Autodesk Inventor part; units mm, degrees
ref_plane "YZ Plane" through (0, 0, 0) normal (1, 0, 0) x (0, 1, 0)
ref_plane "XZ Plane" through (0, 0, 0) normal (0, 1, 0) x (-1, 0, 0)
ref_plane "XY Plane" through (0, 0, 0) normal (0, 0, 1) x (1, 0, 0)
sketch "Sketch1" plane through (0, 0, 0) normal (0, 1, 0) x (-1, 0, 0)
  circle A0 centre (0, 0) radius 3
  circle A1 centre (0, 0) radius 11.049
  circle A2 centre (0, -7.9375) radius 1.27
  circle A3 centre (7.9375, 0) radius 1.27
  circle A4 centre (0, 7.9375) radius 1.27
  circle A5 centre (-7.9375, 0) radius 1.27
  dimension "d4" = 6
  dimension "d6" = 22.098
  dimension "d10" = 2.54
  dimension "d11" = 7.9375
  dimension "d14" = 360
extrude "Extrusion1" add sketch "Sketch1" along normal mid plane 6.35
sketch "Sketch2" plane through (0, 3.175, 0) normal (0, 1, 0) x (1, 0, 0)
  circle A0 centre (0, 0) radius 3
  circle A1 centre (0, 0) radius 4.699
  dimension "d18" = 6
  dimension "d19" = 9.398
extrude "Extrusion2" add sketch "Sketch2" along normal blind 3.175
sketch "Sketch3" plane through (0, -3.175, 0) normal (0, -1, 0) x (1, 0, 0)
  circle A0 centre (0, 0) radius 3
  circle A1 centre (0, 0) radius 4.699
  dimension "d22" = 6
  dimension "d23" = 9.398
extrude "Extrusion3" add sketch "Sketch3" along normal blind 3.175
properties part number "CouplingScrew"
Design review of the part built by this model. Coordinates are the model's own, in mm. A direction names the side the tool comes from. Coordinates: 2 decimals unless noted, no trailing zeros. Order: outer loops, then holes, each group sorted by start corner. A loop starts at its lowest first (then second) coordinate and runs counter-clockwise, first axis right, second up. Notation, with made-up numbers: M -23.5,88 L 5.5,88 A11 cw 5.5,92 Z; hole C 31.25,76 d2. An arc over 180 degrees is marked long. Answer as a JSON object with one key per item and string values. Group by question number.
1) For pin 1 (1 mm diameter, centred on y = 4.5, z = -1, fed in from -X); pin 2 (2 mm diameter, centred on x = 2, y = 1, fed in from +Z); pin 3 (1.5 mm diameter, centred on x = 7.94, z = 0, fed in from +Y); pin 4 (1.5 mm diameter, centred on y = -2, z = -2, fed in from +X), all flat-tipped, find the tip position at first contact; note any pin that passes through.
2) Add section A-A, the plane z = 0. Count the separate pieces of the cut face and the enclosed holes in it, then the cut area to 3 significant figures.
3) Mouldability with a two-part tool opening along Z and no side actions: class faces 1 (the cylindrical face through (1.438, 0.044, 10.955)), 2 (the cylindrical face through (0.28, 0.04, 6.7)), 3 (the flat face through (3, 6.35, 1)) as pulls with the +Z half, pulls with the -Z half, needs draft (parallel to the pull), parting line crosses it, or undercut.
4) Tool access review of faces 4 (the flat face through (0, -3.175, -5)), 5 (the cylindrical face through (-9.11, -0.04, 0.49)), 6 (the cylindrical face through (-0.61, 4.74, 4.66)): name each direction out of +Z, -Z, +X, -X, +Y, -Y from which nothing blocks a thin tool from reaching the whole face with its end or side.
5) Add section D-D, the plane y = 1. Write out the cut boundary in (x, z).
6) Add section C-C, the plane x = -7. Write out the cut boundary in (y, z) (3 decimals), then the cut area to 3 significant figures.
7) Wall thickness on L1, parallel to Z at x = 0, y = 2.05; L2, parallel to Z at x = 0, y = -5.65; L3, parallel to Y at x = 1, z = -9 (3 decimals): over which ranges is each line inside the solid? List them lowest first.
Computed values:
{
 "1": {"pin 1": "stops at x = -4.67", "pin 2": "stops at z = 11", "pin 3": "passes through", "pin 4": "stops at x = 10.98"},
 "2": {"separate pieces": "4", "enclosed holes": "0", "area": "91.5 mm^2"},
 "3": {"face 1": "parting line crosses it", "face 2": "undercut", "face 3": "needs draft"},
 "4": {"face 4": "-Y", "face 5": "+Y, -Y", "face 6": "+Y"},
 "5": {"outline": "C 0,0 d22.1; hole C -7.94,0 d2.54; hole C 0,0 d6; hole C 0,-7.94 d2.54; hole C 0,7.94 d2.54; hole C 7.94,0 d2.54"},
 "6": {"outline": "M -3.175,-8.549 L 3.175,-8.549 L 3.175,-0.857 L -3.175,-0.857 Z; M -3.175,0.857 L 3.175,0.857 L 3.175,8.549 L -3.175,8.549 Z", "area": "97.7 mm^2"},
 "7": {"L1": "z = -11.05 to -9.21, -6.67 to -3, 3 to 6.67, 9.21 to 11.05", "L2": "z = -4.7 to -3, 3 to 4.7", "L3": "y = -3.175 to 3.175"}
}
